```python
from build123d import *

# Parameters (mm, degrees)
SKETCH_1_W      = 90
SKETCH_1_H      = 170
SKETCH_1_W_2    = 27
SKETCH_1_H_2    = 4
EXTRUDE_1_DEPTH = 2


with BuildPart() as part:
    # 草图1 → 凸台-拉伸1 (new body)
    with BuildSketch(Plane(origin=(0, 0, 0), x_dir=(1, 0, 0), z_dir=(0, 1, 0))):
        Rectangle(SKETCH_1_W, SKETCH_1_H)
        Polygon((-29, -66), (-29, -62.731088435), (-25, -62.731088435), (-25, -66), (-22, -66), (-22, -70), (-25, -70), (-25, -72.731088435), (-29, -72.731088435), (-29, -70), (-32, -70), (-32, -66), align=None, mode=Mode.SUBTRACT)
        Polygon((29, -72.731088435), (29, -70), (32, -70), (32, -66), (29, -66), (29, -62.731088435), (25, -62.731088435), (25, -66), (22, -66), (22, -70), (25, -70), (25, -72.731088435), align=None, mode=Mode.SUBTRACT)
        Polygon((25, 72.731088435), (29, 72.731088435), (29, 70), (32, 70), (32, 66), (29, 66), (29, 62.731088435), (25, 62.731088435), (25, 66), (22, 66), (22, 70), (25, 70), align=None, mode=Mode.SUBTRACT)
        Polygon((-29, 72.731088435), (-29, 70), (-32, 70), (-32, 66), (-29, 66), (-29, 62.731088435), (-25, 62.731088435), (-25, 66), (-22, 66), (-22, 70), (-25, 70), (-25, 72.731088435), align=None, mode=Mode.SUBTRACT)
        Polygon((35, -80), (38, -80), (38, -76), (32, -76), (32, -80), align=None, mode=Mode.SUBTRACT)
        Polygon((-32, -76), (-32, -80), (-35, -80), (-38, -80), (-38, -76), align=None, mode=Mode.SUBTRACT)
        Polygon((32, 76), (32, 80), (35, 80), (38, 80), (38, 76), align=None, mode=Mode.SUBTRACT)
        Polygon((-38, 76), (-32, 76), (-32, 80), (-35, 80), (-38, 80), align=None, mode=Mode.SUBTRACT)
        with Locations((0, 57)):
            Rectangle(SKETCH_1_W_2, SKETCH_1_H_2, mode=Mode.SUBTRACT)
        with Locations((0, -57)):
            Rectangle(SKETCH_1_W_2, SKETCH_1_H_2, mode=Mode.SUBTRACT)
    extrude(amount=EXTRUDE_1_DEPTH)


solid = part.part
```
Source: CAD feature listing. Evaluate the final solid. Frame: model axes, mm. Coordinates: 2 decimals unless noted, no trailing zeros. Write each loop counter-clockwise with the first axis right and the second up, starting at its lowest first coordinate (ties: lowest second). Pieces come first, ordered by that corner, then holes. Notation, with made-up numbers: (-25, -17) - (-20, -17) arc R13 cw to (-20, -13) - close; hole circle Ø6 at (-5.5, 31.25). An arc over 180 degrees is marked (long way). Answer as a JSON object with one key per item and string values.
Q1. Material intervals for line 1 (Z direction, x = -8.5, y = 1.4); line 2 (Z direction, x = -24, y = 1.95); line 3 (X direction, y = 1.5, z = 64.5), sorted ascending. Write a range as [from, to].
Ans:
{"line 1": "z = [-85, -59], [-55, 55], [59, 85]", "line 2": "z = [-85, -70], [-66, 66], [70, 85]", "line 3": "x = [-45, -29], [-25, 25], [29, 45]"}
Q2. Section query A-A, the plane x = 34. Output: boundary loops of the cut face in (y, z), plus the area to 3 significant figures.
Ans:
{"outline": "(0, -85) - (2, -85) - (2, -80) - (0, -80) - close; (0, -76) - (2, -76) - (2, 76) - (0, 76) - close; (0, 80) - (2, 80) - (2, 85) - (0, 85) - close", "area": "324 mm2"}
Q3. Section query B-B, the plane y = 1.6. State how many separate pieces and enclosed holes the cut face has, plus the area to 3 significant figures.
Ans:
{"separate pieces": "1", "enclosed holes": "10", "area": "14,700 mm2"}
